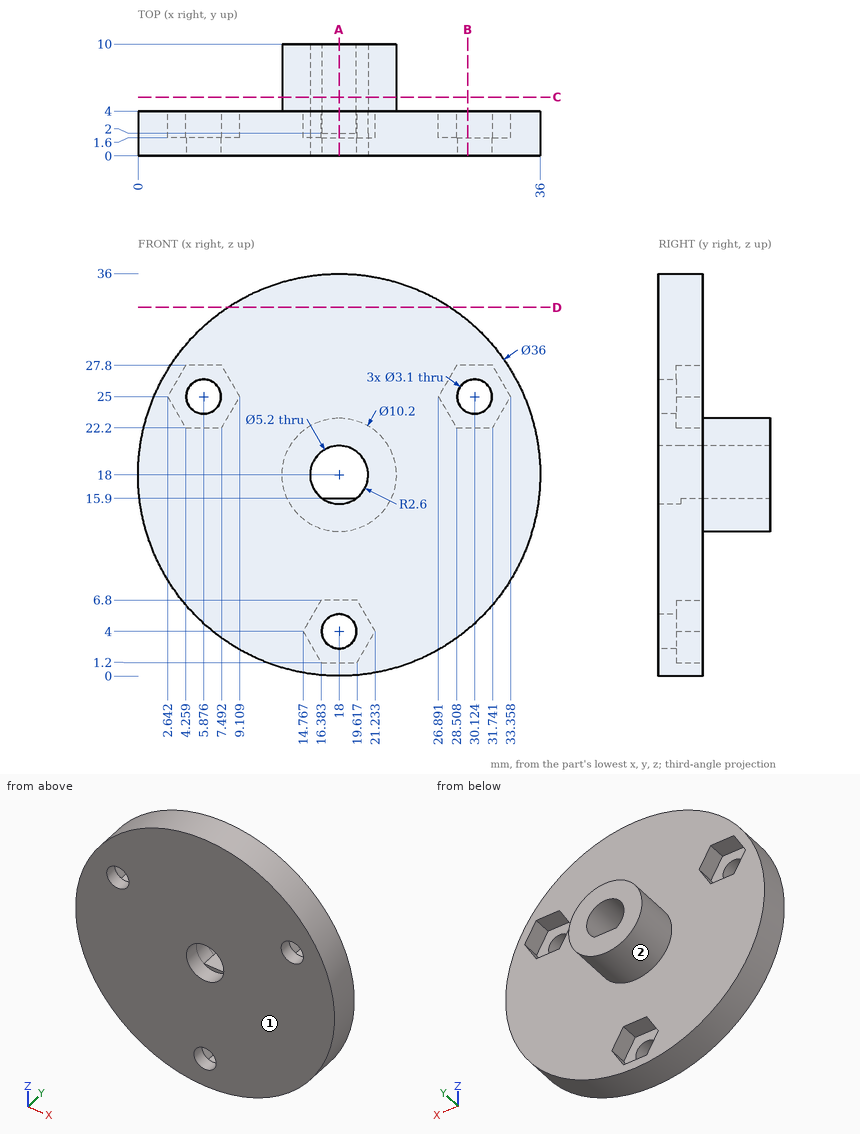
Design review of the part shown in the three views and the two pictorial views. Dimensions are in mm from the part's minimum x, y and z. A direction names the side the tool comes from. Round coordinates to 2 decimals unless told otherwise and drop trailing zeros. Write each loop counter-clockwise with the first axis right and the second up, starting at its lowest first coordinate (ties: lowest second). Pieces come first, ordered by that corner, then holes. Notation, with made-up numbers: (81.5, 13) - (114.5, 13) arc R31 ccw to (114.5, 38) - close; hole circle Ø5 at (74, -36). An arc over 180 degrees is marked (long way). Write item = value, one per line. Start each with the question number.
1. Consider section A-A on x = 18. State the section outline as (y, z) points, plus the area to 3 significant figures.
2. For pin 1 Ø1.9 at (x, y) = (29.5, 3) entering from -Z (1 decimal); pin 2 Ø3 at (x, y) = (22, 1.5) entering from -Z (1 decimal); pin 3 Ø3 at (x, z) = (18, 4) entering from -Y; pin 4 Ø1.7 at (x, z) = (18, 2.5) entering from +Y, all flat-tipped, find the tip position at first contact; note any pin that passes through.
3. Consider section B-B on x = 29.5. State the section outline as (y, z) points.
4. Consider section C-C on y = 5.25. State the section outline as (x, z) points.
5. Consider section D-D on z = 33. State the section outline as (x, y) points.
6. For the marked faces 1 and 2, list the 3-axis set-ups (+Z, -Z, +X, -X, +Y, -Y) from which the entire face can be reached by the end or side of a thin tool; tool diameter is ignored.
7. Wall thickness on L1, parallel to X at y = 6.6, z = 18; L2, parallel to X at y = 0.9, z = 25 (1 decimal); L3, parallel to X at y = 1.55, z = 18: over which ranges is each line inside the solid? List them lowest first.
Evaluation:
q1.outline = (0, 0) - (4, 0) - (4, 1.2) - (1.6, 1.2) - (1.6, 2.45) - (0, 2.45) - close; (0, 5.55) - (1.6, 5.55) - (1.6, 6.8) - (4, 6.8) - (4, 12.9) - (10, 12.9) - (10, 15.9) - (2, 15.9) - (2, 15.4) - (0, 15.4) - close; (0, 20.6) - (10, 20.6) - (10, 23.1) - (4, 23.1) - (4, 36) - (0, 36) - close
q1.area = 139 mm2
q2.pin_1 = 3.4
q2.pin_2 = 0.2
q2.pin_3 = through
q2.pin_4 = 1.6
q3.outline = (0, 4.15) - (4, 4.15) - (4, 22.2) - (1.6, 22.2) - (1.6, 23.58) - (0, 23.58) - close; (0, 26.42) - (1.6, 26.42) - (1.6, 27.8) - (4, 27.8) - (4, 31.85) - (0, 31.85) - close
q4.outline = circle Ø10.2 at (18, 18); hole (16.47, 15.9) - (19.53, 15.9) arc R2.6 ccw (long way) to start
q5.outline = (8.05, 0) - (27.95, 0) - (27.95, 4) - (8.05, 4) - close
q6.face_1 = +Z, -Z, +X, -X, -Y
q6.face_2 = +Y
q7.L1 = 12.9 to 15.4, 20.6 to 23.1
q7.L2 = 1.4 to 4.3, 7.4 to 28.6, 31.7 to 34.6
q7.L3 = 0 to 15.4, 20.6 to 36
